```python
from build123d import *

# Parameters (mm, degrees)
F0_W     = 3.4663490951
F0_H     = 3.8823140785
F0_H_2   = 2.9117353261
F0_H_3   = 0.9705787525
F1_DEPTH = 5
F2_DEPTH = 30
F3_DEPTH = 38.19281
F4_R     = 9.3059115505
F5_DEPTH = 4.488162903


with BuildPart() as f1:
    # F0 (on Top) → F1 (new body)
    with BuildSketch(Plane.XY):
        Polygon((20, -20), (20, 15.512837097), (17.0732010156, 15.512837097), (17.0732010156, 14.5422583446), (13.6068519205, 14.5422583446), (13.6068519205, 15.512837097), (-13.6068519205, 15.512837097), (-13.6068519205, 14.5422583446), (-17.0732010156, 14.5422583446), (-17.0732010156, 15.512837097), (-20, 15.512837097), (-20, -20), align=None)
        with Locations((-15.340026468, -16.4834153838)):
            Rectangle(F0_W, F0_H, mode=Mode.SUBTRACT)
        with Locations((15.340026468, -16.4834153838)):
            Rectangle(F0_W, F0_H, mode=Mode.SUBTRACT)
        Polygon((20, 15.512837097), (20, 20), (-20, 20), (-20, 15.512837097), (-17.0732010156, 15.512837097), (-17.0732010156, 18.4245724231), (-13.6068519205, 18.4245724231), (-13.6068519205, 15.512837097), (13.6068519205, 15.512837097), (13.6068519205, 18.4245724231), (17.0732010156, 18.4245724231), (17.0732010156, 15.512837097), align=None)
        with Locations((15.340026468, -16.4834153838)):
            Rectangle(F0_W, F0_H)
        with Locations((-15.340026468, -16.4834153838)):
            Rectangle(F0_W, F0_H)
        with Locations((15.340026468, 16.9687047601)):
            Rectangle(F0_W, F0_H_2)
        with Locations((-15.340026468, 16.9687047601)):
            Rectangle(F0_W, F0_H_2)
        with Locations((15.340026468, 15.0275477208)):
            Rectangle(F0_W, F0_H_3)
        with Locations((-15.340026468, 15.0275477208)):
            Rectangle(F0_W, F0_H_3)
    extrude(amount=F1_DEPTH)

    # F0 (on Top) → F2 (join)
    with BuildSketch(Plane.XY):
        with Locations((15.340026468, -16.4834153838)):
            Rectangle(F0_W, F0_H)
        with Locations((-15.340026468, -16.4834153838)):
            Rectangle(F0_W, F0_H)
        with Locations((-15.340026468, 16.9687047601)):
            Rectangle(F0_W, F0_H_2)
        with Locations((15.340026468, 16.9687047601)):
            Rectangle(F0_W, F0_H_2)
        with Locations((15.340026468, 15.0275477208)):
            Rectangle(F0_W, F0_H_3)
        with Locations((-15.340026468, 15.0275477208)):
            Rectangle(F0_W, F0_H_3)
    extrude(amount=-F2_DEPTH)

    # F0 (on Top) → F3 (join)
    with BuildSketch(Plane.XY):
        Polygon((20, 15.512837097), (20, 20), (-20, 20), (-20, 15.512837097), (-17.0732010156, 15.512837097), (-17.0732010156, 18.4245724231), (-13.6068519205, 18.4245724231), (-13.6068519205, 15.512837097), (13.6068519205, 15.512837097), (13.6068519205, 18.4245724231), (17.0732010156, 18.4245724231), (17.0732010156, 15.512837097), align=None)
        with Locations((-15.340026468, 16.9687047601)):
            Rectangle(F0_W, F0_H_2)
        with Locations((15.340026468, 16.9687047601)):
            Rectangle(F0_W, F0_H_2)
    extrude(amount=F3_DEPTH)

    # F4 (on face) → F5 (cut, through all)
    with BuildSketch(Plane.XZ.offset(-15.512837097)):
        with Locations((0, 23.2225228101)):
            Circle(F4_R)
    extrude(amount=-F5_DEPTH, mode=Mode.SUBTRACT)


solid = f1.part
```
Can you work these out from the model? Positions are in its coordinate system, mm. A direction names the side the tool comes from. Give positions to 0.01 mm unless a question says otherwise; leave off trailing zeros. Order: outer loops, then holes, each group sorted by start corner. A loop starts at its lowest first (then second) coordinate and runs counter-clockwise, first axis right, second up. Notation, with made-up numbers: M 65.25,1.5 L 124.25,1.5 A15 cw 124.25,20.5 Z; hole C 13.5,20 d9. An arc over 180 degrees is marked long. Write item = value, one per line. Start each with the question number.
Q1. Suppose I cut it at C-C (z = 31.5). Write out the boundary of the cut face in (x, y).
Q2. For faces 4 (the flat face through (15, -14.542, -15)), 5 (the flat face through (-17.073, 17, -15)), 6 (the flat face through (0, -2, 5)), which set-ups out of +Z, -Z, +X, -X, +Y, -Y let a thin tool reach every point of the face, with its end or its side?
Q3. Suppose I cut it at A-A (x = 0). Write out the boundary of the cut face in (y, z).
Q4. I need wall thicknesses on probe 1 along Z at (x, y) = (0, 17.4); probe 2 along Y at (x, z) = (-14.5, -13.5); probe 3 along Z at (x, y) = (-7, -7). Which ranges of each line are inside material? Lowest first, please. Write a range as [from, to].
Q5. Suppose I cut it at D-D (x = -5). Write out the boundary of the cut face in (y, z).
Q6. We'd pull the mould along X, two halves only. Please class faces 1 (the flat face through (13.607, -17, -15)), 2 (the flat face through (-15, -16, -30)), 3 (the flat face through (-17.073, -17, -15)): pulls with the +X half, pulls with the -X half, needs draft (parallel to the pull), parting line crosses it, or undercut.
Q7. Suppose I cut it at B-B (y = -16.5). Write out the boundary of the cut face in (x, z).
Q8. Will these pins go through, and if not, where does the flat tip stop? pin 1 Ø4 at (x, y) = (0, -11.5) entering from +Z; pin 2 Ø4.5 at (y, z) = (-17, -12.5) entering from -X; pin 3 Ø1 at (x, z) = (16, -18.5) entering from -Y.
Check result:
q1.outline = M -20,15.51 L -4.25,15.51 L -4.25,20 L -20,20 Z; M 4.25,15.51 L 20,15.51 L 20,20 L 4.25,20 Z
q2.face_4 = -Z, +X, -X
q2.face_5 = -Z, -X, +Y, -Y
q2.face_6 = +Z, +X, -X, -Y
q3.outline = M -20,0 L 20,0 L 20,13.92 L 15.51,13.92 L 15.51,5 L -20,5 Z; M 15.51,32.53 L 20,32.53 L 20,38.19 L 15.51,38.19 Z
q4.probe_1 = [0, 13.92], [32.53, 38.19]
q4.probe_2 = [-18.42, -14.54], [14.54, 18.42]
q4.probe_3 = [0, 5]
q5.outline = M -20,0 L 20,0 L 20,15.37 L 15.51,15.37 L 15.51,5 L -20,5 Z; M 15.51,31.07 L 20,31.07 L 20,38.19 L 15.51,38.19 Z
q6.face_1 = undercut
q6.face_2 = needs draft
q6.face_3 = pulls with the -X half
q7.outline = M -20,0 L -17.07,0 L -17.07,-30 L -13.61,-30 L -13.61,0 L 13.61,0 L 13.61,-30 L 17.07,-30 L 17.07,0 L 20,0 L 20,5 L -20,5 Z
q8.pin_1 = 5
q8.pin_2 = -17.07
q8.pin_3 = -18.42
